Read the model definition and answer for the solid it produces. Units are mm, in the model's axes. A direction names the side the tool comes from. Round coordinates to 2 decimals unless told otherwise and drop trailing zeros. Loops run counter-clockwise (first coordinate to the right, second up) from the corner with the lowest first, then second, coordinate; pieces in that order, holes last. Notation, with made-up numbers: (5, -9) -> (27, -9) arc R30 ccw to (27, 24) -> close; hole circle Ø4 at (43.5, 80.5). An arc over 180 degrees is marked (long way). Put each result on its own line as item: value.
from build123d import *

# Parameters (mm, degrees)
F0_R        = 30
F1_DEPTH    = 3
F4_DEPTH    = 1.5
F5_T1_DEPTH = 9.1064563612
F2_R        = 1.5
F3_DEPTH    = 2
F6_DEPTH    = 25


# Not quite as in the source:
# - a fillet or chamfer that OpenCascade refuses, or shapes differently, is made with other operations: its cross-section is extruded or revolved along the edge and cut away or added


with BuildPart() as f1:
    # F0 (on Front) → F1 (new body)
    with BuildSketch(Plane.XZ):
        Circle(F0_R)
        with BuildLine():
            ThreePointArc((0, 16.4), (11.5965512115, 11.5965512115), (16.4, 0))
            ThreePointArc((16.4, 0), (11.5965511405, -11.5965512824), (-2.007e-07, -16.4))
            ThreePointArc((-2.007e-07, -16.4), (-11.5965512889, -11.596551134), (-16.4, 1.83e-08))
            ThreePointArc((-16.4, 1.83e-08), (-11.596551205, 11.5965512179), (0, 16.4))
        make_face(mode=Mode.SUBTRACT)
        with BuildLine():
            ThreePointArc((7.6903565933, 7.6903565933), (12.3769167702, 6.7950416767), (15.650867052, 3.3242082546))
            ThreePointArc((15.650867052, 3.3242082546), (11.313708499, 11.313708499), (3.3242082546, 15.650867052))
            ThreePointArc((3.3242082546, 15.650867052), (6.5507676639, 12.7912489678), (7.75, 8.65))
            ThreePointArc((7.75, 8.65), (7.7350747766, 8.1692524561), (7.6903565933, 7.6903565933))
        make_face()
        with BuildLine():
            ThreePointArc((3.3242082546, -15.650867052), (11.313708499, -11.313708499), (15.650867052, -3.3242082546))
            ThreePointArc((15.650867052, -3.3242082546), (12.3769167702, -6.7950416767), (7.6903565933, -7.6903565933))
            ThreePointArc((7.6903565933, -7.6903565933), (7.7350747766, -8.1692524561), (7.75, -8.65))
            ThreePointArc((7.75, -8.65), (6.5507676639, -12.7912489678), (3.3242082546, -15.650867052))
        make_face()
        with BuildLine():
            ThreePointArc((-7.6903565933, 7.6903565933), (-6.7950416767, 12.3769167702), (-3.3242082546, 15.650867052))
            ThreePointArc((-3.3242082546, 15.650867052), (-11.313708499, 11.313708499), (-15.650867052, 3.3242082546))
            ThreePointArc((-15.650867052, 3.3242082546), (-12.3769167702, 6.7950416767), (-7.6903565933, 7.6903565933))
        make_face()
        with BuildLine():
            ThreePointArc((-15.650867052, -3.3242082546), (-11.313708499, -11.313708499), (-3.3242082546, -15.650867052))
            ThreePointArc((-3.3242082546, -15.650867052), (-6.7950416767, -12.3769167702), (-7.6903565933, -7.6903565933))
            ThreePointArc((-7.6903565933, -7.6903565933), (-12.3769167702, -6.7950416767), (-15.650867052, -3.3242082546))
        make_face()
        with BuildLine():
            ThreePointArc((15.650867052, 3.3242082546), (16.2103974649, 1.7037870094), (16.4, 0))
            ThreePointArc((16.4, 0), (11.5965512115, 11.5965512115), (0, 16.4))
            ThreePointArc((0, 16.4), (1.7037870094, 16.2103974649), (3.3242082546, 15.650867052))
            ThreePointArc((3.3242082546, 15.650867052), (11.313708499, 11.313708499), (15.650867052, 3.3242082546))
        make_face()
        with BuildLine():
            ThreePointArc((-2.007e-07, -16.4), (11.5965511405, -11.5965512824), (16.4, 0))
            ThreePointArc((16.4, 0), (16.2103974649, -1.7037870094), (15.650867052, -3.3242082546))
            ThreePointArc((15.650867052, -3.3242082546), (11.313708499, -11.313708499), (3.3242082546, -15.650867052))
            ThreePointArc((3.3242082546, -15.650867052), (1.7037869115, -16.2103974869), (-2.007e-07, -16.4))
        make_face()
        with BuildLine():
            ThreePointArc((-3.3242082546, 15.650867052), (-1.7037870094, 16.2103974649), (0, 16.4))
            ThreePointArc((0, 16.4), (-11.596551205, 11.5965512179), (-16.4, 1.83e-08))
            ThreePointArc((-16.4, 1.83e-08), (-16.2103974628, 1.7037870183), (-15.650867052, 3.3242082546))
            ThreePointArc((-15.650867052, 3.3242082546), (-11.313708499, 11.313708499), (-3.3242082546, 15.650867052))
        make_face()
        with BuildLine():
            ThreePointArc((-16.4, 1.83e-08), (-11.5965512889, -11.596551134), (-2.007e-07, -16.4))
            ThreePointArc((-2.007e-07, -16.4), (-1.7037871073, -16.2103974428), (-3.3242082546, -15.650867052))
            ThreePointArc((-3.3242082546, -15.650867052), (-11.313708499, -11.313708499), (-15.650867052, -3.3242082546))
            ThreePointArc((-15.650867052, -3.3242082546), (-16.2103974669, -1.7037870005), (-16.4, 1.83e-08))
        make_face()
    extrude(amount=F1_DEPTH)

    # F0 (on Front) → F4 (join)
    with BuildSketch(Plane.XZ):
        with BuildLine():
            ThreePointArc((7.6903565933, 7.6903565933), (12.3769167702, 6.7950416767), (15.650867052, 3.3242082546))
            ThreePointArc((15.650867052, 3.3242082546), (11.313708499, 11.313708499), (3.3242082546, 15.650867052))
            ThreePointArc((3.3242082546, 15.650867052), (6.5507676639, 12.7912489678), (7.75, 8.65))
            ThreePointArc((7.75, 8.65), (7.7350747766, 8.1692524561), (7.6903565933, 7.6903565933))
        make_face()
        with BuildLine():
            ThreePointArc((3.3242082546, -15.650867052), (11.313708499, -11.313708499), (15.650867052, -3.3242082546))
            ThreePointArc((15.650867052, -3.3242082546), (12.3769167702, -6.7950416767), (7.6903565933, -7.6903565933))
            ThreePointArc((7.6903565933, -7.6903565933), (7.7350747766, -8.1692524561), (7.75, -8.65))
            ThreePointArc((7.75, -8.65), (6.5507676639, -12.7912489678), (3.3242082546, -15.650867052))
        make_face()
        with BuildLine():
            ThreePointArc((-7.6903565933, 7.6903565933), (-6.7950416767, 12.3769167702), (-3.3242082546, 15.650867052))
            ThreePointArc((-3.3242082546, 15.650867052), (-11.313708499, 11.313708499), (-15.650867052, 3.3242082546))
            ThreePointArc((-15.650867052, 3.3242082546), (-12.3769167702, 6.7950416767), (-7.6903565933, 7.6903565933))
        make_face()
        with BuildLine():
            ThreePointArc((-15.650867052, -3.3242082546), (-11.313708499, -11.313708499), (-3.3242082546, -15.650867052))
            ThreePointArc((-3.3242082546, -15.650867052), (-6.7950416767, -12.3769167702), (-7.6903565933, -7.6903565933))
            ThreePointArc((-7.6903565933, -7.6903565933), (-12.3769167702, -6.7950416767), (-15.650867052, -3.3242082546))
        make_face()
    extrude(amount=-F4_DEPTH)

    # F5: fillet of radius 0.5 on 8 edges, made by hand

    # F5_s2 → F5_t1 (cut)
    with BuildSketch(Plane.XZ.offset(-9.1064563612)):
        with BuildLine():
            ThreePointArc((-6.2268118052, -14.738616446), (-5.6223691009, -14.5644243012), (-5.6666346068, -13.936941671))
            ThreePointArc((-5.6666346068, -13.936941671), (-4.5763739896, -14.9045424379), (-3.3242082546, -15.650867052))
            ThreePointArc((-3.3242082546, -15.650867052), (-4.7972436187, -15.263893791), (-6.2268118052, -14.738616446))
        make_face()
        with BuildLine():
            ThreePointArc((6.2268118052, -14.738616446), (5.6223691009, -14.5644243012), (5.6666346068, -13.936941671))
            ThreePointArc((5.6666346068, -13.936941671), (4.5763739896, -14.9045424379), (3.3242082546, -15.650867052))
            ThreePointArc((3.3242082546, -15.650867052), (4.7972436187, -15.263893791), (6.2268118052, -14.738616446))
        make_face()
        with BuildLine():
            ThreePointArc((13.936941671, 5.6666346068), (14.5644243012, 5.6223691009), (14.738616446, 6.2268118052))
            ThreePointArc((14.738616446, 6.2268118052), (15.263893791, 4.7972436187), (15.650867052, 3.3242082546))
            ThreePointArc((15.650867052, 3.3242082546), (14.9045424379, 4.5763739896), (13.936941671, 5.6666346068))
        make_face()
        with BuildLine():
            ThreePointArc((13.936941671, -5.6666346068), (14.5644243012, -5.6223691009), (14.738616446, -6.2268118052))
            ThreePointArc((14.738616446, -6.2268118052), (15.263893791, -4.7972436187), (15.650867052, -3.3242082546))
            ThreePointArc((15.650867052, -3.3242082546), (14.9045424379, -4.5763739896), (13.936941671, -5.6666346068))
        make_face()
        with BuildLine():
            ThreePointArc((-13.936941671, 5.6666346068), (-14.5644243012, 5.6223691009), (-14.738616446, 6.2268118052))
            ThreePointArc((-14.738616446, 6.2268118052), (-15.263893791, 4.7972436187), (-15.650867052, 3.3242082546))
            ThreePointArc((-15.650867052, 3.3242082546), (-14.9045424379, 4.5763739896), (-13.936941671, 5.6666346068))
        make_face()
        with BuildLine():
            ThreePointArc((-14.738616446, -6.2268118052), (-14.5644243012, -5.6223691009), (-13.936941671, -5.6666346068))
            ThreePointArc((-13.936941671, -5.6666346068), (-14.9045424379, -4.5763739896), (-15.650867052, -3.3242082546))
            ThreePointArc((-15.650867052, -3.3242082546), (-15.263893791, -4.7972436187), (-14.738616446, -6.2268118052))
        make_face()
        with BuildLine():
            ThreePointArc((6.2268118052, 14.738616446), (5.6223691009, 14.5644243012), (5.6666346068, 13.936941671))
            ThreePointArc((5.6666346068, 13.936941671), (4.5763739896, 14.9045424379), (3.3242082546, 15.650867052))
            ThreePointArc((3.3242082546, 15.650867052), (4.7972436187, 15.263893791), (6.2268118052, 14.738616446))
        make_face()
        with BuildLine():
            ThreePointArc((-6.2268118052, 14.738616446), (-5.6223691009, 14.5644243012), (-5.6666346068, 13.936941671))
            ThreePointArc((-5.6666346068, 13.936941671), (-4.5763739896, 14.9045424379), (-3.3242082546, 15.650867052))
            ThreePointArc((-3.3242082546, 15.650867052), (-4.7972436187, 15.263893791), (-6.2268118052, 14.738616446))
        make_face()
    extrude(amount=F5_T1_DEPTH, mode=Mode.SUBTRACT)

    # F2 (on face) → F3 (cut)
    with BuildSketch(Plane.XZ.offset(3)):
        Polygon((-15.0011106999, 10.9), (-11.9988893001, 10.9), (-10.4977786002, 13.5), (-11.9988893001, 16.1), (-15.0011106999, 16.1), (-16.5022213998, 13.5), align=None)
        with Locations((-13.5, 13.5)):
            Circle(F2_R, mode=Mode.SUBTRACT)
        Polygon((11.9988893001, 10.9), (15.0011106999, 10.9), (16.5022213998, 13.5), (15.0011106999, 16.1), (11.9988893001, 16.1), (10.4977786002, 13.5), align=None)
        with Locations((13.5, 13.5)):
            Circle(F2_R, mode=Mode.SUBTRACT)
        Polygon((-11.9988893001, -10.9), (-15.0011106999, -10.9), (-16.5022213998, -13.5), (-15.0011106999, -16.1), (-11.9988893001, -16.1), (-10.4977786002, -13.5), align=None)
        with Locations((-13.5, -13.5)):
            Circle(F2_R, mode=Mode.SUBTRACT)
        Polygon((15.0011106999, -10.9), (11.9988893001, -10.9), (10.4977786002, -13.5), (11.9988893001, -16.1), (15.0011106999, -16.1), (16.5022213998, -13.5), align=None)
        with Locations((13.5, -13.5)):
            Circle(F2_R, mode=Mode.SUBTRACT)
    extrude(amount=-F3_DEPTH, mode=Mode.SUBTRACT)

    # F2 (on face) → F6 (cut)
    with BuildSketch(Plane.XZ.offset(3)):
        with Locations((-13.5, 13.5)):
            Circle(F2_R)
        with Locations((13.5, 13.5)):
            Circle(F2_R)
        with Locations((13.5, -13.5)):
            Circle(F2_R)
        with Locations((-13.5, -13.5)):
            Circle(F2_R)
    extrude(amount=-F6_DEPTH, mode=Mode.SUBTRACT)


solid = f1.part
Item 1: The part is cut by section C-C (x = -2). Determine the outline of the cut face in (y, z), then the cut area to 3 significant figures.
Derived:
outline: (-3, -29.93) -> (0, -29.93) -> (0, -16.14) -> (-3, -16.14) -> close; (-3, 16.14) -> (0, 16.14) -> (0, 29.93) -> (-3, 29.93) -> close
area: 82.8 mm^2
Item 2: For a pull along Z with two mould halves and no side action, classify faces 1 (the flat face through (-15.762, -2.014, 12.218)), 2 (the flat face through (13, -3, 7)) as pulls with the +Z half, pulls with the -Z half, needs draft (parallel to the pull), parting line crosses it, or undercut.
Derived:
face 1: undercut
face 2: needs draft
Item 3: The part is cut by section B-B (x = 13). Determine the outline of the cut face in (y, z), then the cut area to 3 significant figures.
Derived:
outline: (-3, -27.04) -> (0, -27.04) -> (0, -14.91) -> (-1, -14.91) -> (-1, -16.1) -> (-3, -16.1) -> close; (-3, -10.9) -> (-1, -10.9) -> (-1, -12.09) -> (0, -12.09) -> (0, -9.33) -> (1.5, -9.33) -> (1.5, -6.41) -> (-3, -6.41) -> close; (-3, 6.41) -> (1.5, 6.41) -> (1.5, 9.33) -> (0, 9.33) -> (0, 12.09) -> (-1, 12.09) -> (-1, 10.9) -> (-3, 10.9) -> close; (-3, 16.1) -> (-1, 16.1) -> (-1, 14.91) -> (0, 14.91) -> (0, 27.04) -> (-3, 27.04) -> close
area: 106 mm^2
Item 4: Which of the six approach directions +Z, -Z, +X, -X, +Y, -Y give full straight-line access (tool end or side, diameter ignored) to faces 3 (the cylindrical face through (-15, -0.51, -13.43)), 4 (the flat face through (20, 0, 0)), 5 (the flat face through (11.238, -2.014, -14.782))?
Derived:
face 3: +Y, -Y
face 4: +Y
face 5: -Y
Item 5: The part is cut by section A-A (z = 1.5). Determine the outline of the cut face in (x, y), then the cut area to 3 significant figures.
Derived:
outline: (-29.96, -3) -> (-16.25, -3) -> (-16.25, 0) -> (-29.96, 0) -> close; (16.25, -3) -> (29.96, -3) -> (29.96, 0) -> (16.25, 0) -> close
area: 82.3 mm^2
Item 6: The part is cut by section D-D (z = 25.5). Determine the outline of the cut face in (x, y).
Derived:
outline: (-15.8, -3) -> (15.8, -3) -> (15.8, 0) -> (-15.8, 0) -> close
Item 7: Flat-ended cylindrical pins translate along their axes: pin 1 Ø1.6 at (x, z) = (12, 13.5) entering from -Y; pin 2 Ø2.5 at (x, z) = (-13.5, -13.5) entering from +Y; pin 3 Ø4 at (x, z) = (-13.5, 13.5) entering from +Y; pin 4 Ø1 at (x, y) = (13.5, -2) entering from -Z. Find the tip coordinate at first contact, or state that the pin passes through.
Derived:
pin 1: stops at y = -1
pin 2: passes through
pin 3: stops at y = 0
pin 4: stops at z = -27.04
Item 8: Find the intervals of material crossed by line 1 along Z through (x, y) = (13, -2.6); line 2 along Z through (x, y) = (13.5, -0.75); line 3 along X through (y, z) = (-0.6, 14), in increasing order.
Derived:
line 1: z = -27.04 to -16.1, -10.9 to -6.41, 6.41 to 10.9, 16.1 to 27.04
line 2: z = -26.79 to -15, -12 to -6.04, 6.04 to 12, 15 to 26.79
line 3: x = -26.53 to -14.91, -12.09 to -5.61, 5.61 to 12.09, 14.91 to 26.53
